Read the model definition and answer for the solid it produces. Units are mm, in the model's axes. A direction names the side the tool comes from. Coordinates: 2 decimals unless noted, no trailing zeros. Loops run counter-clockwise (first coordinate to the right, second up) from the corner with the lowest first, then second, coordinate; pieces in that order, holes last. Notation, with made-up numbers: (78, 43) -> (88, 43) arc R19 cw to (88, 77) -> close; hole circle Ø4 at (44.25, 29). An arc over 180 degrees is marked (long way). Answer as a JSON object with one key per item and string values. Group by question number.
Q1. The part is cut by section D-D on z = 8.25. Write down the section's boundary in (x, y).
Q2. Straight lines are drawn through the part: line 1 along Z through (x, y) = (0, 1.6); line 2 along Z through (x, y) = (0, 2.25); line 3 along X through (y, z) = (2.2, 9.5). For each, find the intervals that lie inside material, in ascending order. Write a range as [from, to].
Q3. Determine the mould class of faces 5 (the conical face through (-0.115, -5.947, 9.394)), 6 (the flat face through (0, -4, 11.9)), 7 (the flat face through (-1.81, -1.84, 6.08)), 8 (the cylindrical face through (-0.48, 1.77, 8.74)) for opening direction X: released by +X, released by -X, zero draft, split by the parting line, or undercut.
Q4. Each of these flat-tipped pins is pushed along its axis until it touches: P1, Ø3, axis at y = -4.5, z = 8.5, coming from the -X side; P2, Ø1.1, axis at x = 0.5, y = -4.5, coming from the +Z side; P3, Ø1.2, axis at y = -4, z = 9.5, coming from the +X side. Where does it stop, or does it pass through?
Q5. The part is cut by section A-A on y = 0. Write down the section's boundary in (x, z), and give its area (3 significant figures).
Q6. The part is cut by section B-B on z = 4. Write down the section's boundary in (x, y).
Q7. For faces 1 (the flat face through (0, 2, 12)), 2 (the flat face through (-1.1, -4, 9)), 3 (the cylindrical face through (0.12, -3.22, 8.61)), 4 (the flat face through (1.1, -4, 9)), determine the directions among +Z, -Z, +X, -X, +Y, -Y from which every point of the face is accessible in a straight line to the end or side of a thin tool.
Q8. The part is cut by section C-C on x = 1.55. Write down the section's boundary in (y, z), and give its area (3 significant figures).
from build123d import *

# Parameters (mm, degrees)
SKETCH1_W                      = 4.5
SKETCH1_H                      = 5
BOSS_EXTRUDE1_DEPTH            = 12
SKETCH4_R                      = 1.75
BOSS_EXTRUDE3_DEPTH            = 2.5
SKETCH5_R                      = 1.25
CUT_EXTRUDE1_DEPTH             = 15.5
SKETCH7_W                      = 2.2
SKETCH7_H                      = 4.7
BOSS_EXTRUDE4_DEPTH            = 5.8
CUT_EXTRUDE2_DEPTH             = 13
CUT_EXTRUDE6_DEPTH             = 12.9
CUT_EXTRUDE3_DEPTH             = 3.25
CUT_EXTRUDE3_DEPTH_BACK        = 3.25
CUT_EXTRUDE4_DEPTH             = 3.25
CIRPATTERN3_COUNT              = 60
F_1_8_1_8_DIAMETER_HOLE1_D     = 1.8
F_1_8_1_8_DIAMETER_HOLE1_DEPTH = 8.2
F_1_8_1_8_DIAMETER_HOLE1_TIP   = 0.540774557


with BuildPart() as part:
    # Sketch1 → Boss-Extrude1 (new body)
    with BuildSketch(Plane.XY):
        with Locations((0, 0.2)):
            Rectangle(SKETCH1_W, SKETCH1_H)
    extrude(amount=BOSS_EXTRUDE1_DEPTH)

    # Sketch4 → Boss-Extrude3 (add)
    with BuildSketch(Plane.XY.offset(12)):
        Circle(SKETCH4_R)
    extrude(amount=BOSS_EXTRUDE3_DEPTH)

    # Sketch5 → Cut-Extrude1 (cut, through all)
    with BuildSketch(Plane.XY.offset(14.5)):
        Circle(SKETCH5_R)
    extrude(amount=-CUT_EXTRUDE1_DEPTH, mode=Mode.SUBTRACT)

    # Sketch7 → Boss-Extrude4 (add)
    with BuildSketch(Plane.XY.offset(6.1)):
        with Locations((0, -4.65)):
            Rectangle(SKETCH7_W, SKETCH7_H)
    extrude(amount=BOSS_EXTRUDE4_DEPTH)

    # Sketch8 → Cut-Extrude2 (cut, through all)
    with BuildSketch(Plane.XY.offset(12)):
        Polygon((1.35, -2.3), (2.25, -1.4), (2.25, -2.3), align=None)
        Polygon((-1.35, -2.3), (-2.25, -2.3), (-2.25, -1.4), align=None)
    extrude(amount=-CUT_EXTRUDE2_DEPTH, mode=Mode.SUBTRACT)

    # Sketch10 → Cut-Extrude6 (cut, through all)
    with BuildSketch(Plane.XY.offset(11.9)):
        Polygon((-0.638119785, -7), (-1.1, -7), (-1.1, -6.2), align=None)
        Polygon((1.1, -7), (1.1, -6.2), (0.638119785, -7), align=None)
    extrude(amount=-CUT_EXTRUDE6_DEPTH, mode=Mode.SUBTRACT)

    # Sketch9 → Cut-Extrude3 (cut, two sides)
    with BuildSketch(Plane(origin=(0, 0, 0), x_dir=(0, 0, -1), z_dir=(1, 0, 0))) as cut_extrude3_sk:
        with BuildLine():
            Line((-11.9, -6.570266454), (-11.9, -8))
            Line((-11.9, -8), (-6.1, -8))
            Line((-6.1, -8), (-6.1, -6.570266454))
            ThreePointArc((-6.1, -6.570266454), (-9, -7), (-11.9, -6.570266454))
        make_face()
    extrude(amount=CUT_EXTRUDE3_DEPTH, mode=Mode.SUBTRACT)
    extrude(cut_extrude3_sk.sketch, amount=-CUT_EXTRUDE3_DEPTH_BACK, mode=Mode.SUBTRACT)

    # Sketch9<3> → Cut-Extrude4 (cut, symmetric)
    with BuildSketch(Plane(origin=(0, 0, 0), x_dir=(0, 0, -1), z_dir=(1, 0, 0))):
        with BuildLine():
            Line((-8.51191829, -6.98808171), (-9, -6.5))
            Line((-9, -6.5), (-9.48808171, -6.98808171))
            ThreePointArc((-9.48808171, -6.98808171), (-9, -7), (-8.51191829, -6.98808171))
        make_face()
    cut_extrude4 = extrude(amount=CUT_EXTRUDE4_DEPTH, both=True, mode=Mode.SUBTRACT)

    # CirPattern3: Cut-Extrude4 ×60 about axis, 6 skipped
    cirpattern3_axis = Axis((0, 3, 9), (1, 0, 0))
    add([cut_extrude4.rotate(cirpattern3_axis, i * 360 / CIRPATTERN3_COUNT) for i in range(1, CIRPATTERN3_COUNT) if i not in (8, 9, 10, 11, 12, 13)], mode=Mode.SUBTRACT)

    # Ø1.8 (1.8) Diameter Hole1
    with Locations(Plane(origin=(0, 2.7, 0), x_dir=(1, 0, 0), z_dir=(0, 1, 0))):
        with Locations((0, -9.5)):
            Hole(F_1_8_1_8_DIAMETER_HOLE1_D / 2, depth=F_1_8_1_8_DIAMETER_HOLE1_DEPTH)
            with Locations((0, 0, -(F_1_8_1_8_DIAMETER_HOLE1_DEPTH + F_1_8_1_8_DIAMETER_HOLE1_TIP / 2))):  # 118° drill point
                Cone(0, F_1_8_1_8_DIAMETER_HOLE1_D / 2, F_1_8_1_8_DIAMETER_HOLE1_TIP, mode=Mode.SUBTRACT)


solid = part.part
Final values:
{
 "1": {"outline": "(-2.25, -1.4) -> (-1.35, -2.3) -> (-1.1, -2.3) -> (-1.1, -6.2) -> (-0.78, -6.75) -> (0.78, -6.75) -> (1.1, -6.2) -> (1.1, -2.3) -> (1.35, -2.3) -> (2.25, -1.4) -> (2.25, 2.7) -> (-2.25, 2.7) -> close; hole circle Ø2.5 at (0, 0)"},
 "2": {"line 1": "z = [0, 8.6], [10.4, 14.5]", "line 2": "z = [0, 8.6], [10.4, 12]", "line 3": "x = [-2.25, -0.9], [0.9, 2.25]"},
 "3": {"face 5": "undercut", "face 6": "zero draft", "face 7": "released by -X", "face 8": "undercut"},
 "4": {"P1": "stops at x = -1.1", "P2": "stops at z = 11.9", "P3": "stops at x = 1.1"},
 "5": {"outline": "(-2.25, 0) -> (-1.25, 0) -> (-1.25, 14.5) -> (-1.75, 14.5) -> (-1.75, 12) -> (-2.25, 12) -> close; (1.25, 0) -> (2.25, 0) -> (2.25, 12) -> (1.75, 12) -> (1.75, 14.5) -> (1.25, 14.5) -> close", "area": "26.5 mm2"},
 "6": {"outline": "(-2.25, -1.4) -> (-1.35, -2.3) -> (1.35, -2.3) -> (2.25, -1.4) -> (2.25, 2.7) -> (-2.25, 2.7) -> close; hole circle Ø2.5 at (0, 0)"},
 "7": {"face 1": "+Z", "face 2": "+Z, -Z, -X, -Y", "face 3": "+Y", "face 4": "+Z, -Z, +X, -Y"},
 "8": {"outline": "(-2.1, 0) -> (2.7, 0) -> (2.7, 12) -> (0.81, 12) -> (0.81, 14.5) -> (-0.81, 14.5) -> (-0.81, 12) -> (-2.1, 12) -> close", "area": "61.7 mm2"}
}
